```python
from build123d import *

# Parameters (mm, degrees)
SKETCH_2_R          = 2.25
CUT_EXTRUDE_1_DEPTH = 57.577380639
SKETCH_3_R          = 3.75
CUT_EXTRUDE_2_DEPTH = 4


with BuildPart() as part:
    # Эскиз1 → Повернуть1 (revolve)
    with BuildSketch(Plane.XY, mode=Mode.PRIVATE) as revolve_1_sk:
        Polygon((5, 55), (5, 0), (20, 0), (20, 6), (9.5, 6), (9.5, 55), align=None)
    revolve(revolve_1_sk.sketch.rotate(Axis((0, 53.580953173, 0), (0, -1, 0)), 90), axis=Axis((0, 53.580953173, 0), (0, -1, 0)))

    # Эскиз2 → Вырез-Вытянуть1 (cut, through all)
    with BuildSketch(Plane(origin=(0, 6, 0), x_dir=(1, 0, 0), z_dir=(0, 1, 0))):
        with Locations(Location((14.5, 0, 0), (0, 0, 270))):
            Circle(SKETCH_2_R)
        with Locations(Location((0, -14.5, 0), (0, 0, 270))):
            Circle(SKETCH_2_R)
        with Locations(Location((-14.5, 0, 0), (0, 0, 270))):
            Circle(SKETCH_2_R)
        with Locations(Location((0, 14.5, 0), (0, 0, 270))):
            Circle(SKETCH_2_R)
    extrude(amount=-CUT_EXTRUDE_1_DEPTH, mode=Mode.SUBTRACT)

    # Эскиз3 → Вырез-Вытянуть2 (cut)
    with BuildSketch(Plane.XZ):
        with Locations(Location((-14.5, 0, 0), (0, 0, 270))):
            Circle(SKETCH_3_R)
        with Locations(Location((0, 14.5, 0), (0, 0, 270))):
            Circle(SKETCH_3_R)
        with Locations(Location((14.5, 0, 0), (0, 0, 270))):
            Circle(SKETCH_3_R)
        with Locations(Location((0, -14.5, 0), (0, 0, 270))):
            Circle(SKETCH_3_R)
    extrude(amount=-CUT_EXTRUDE_2_DEPTH, mode=Mode.SUBTRACT)


solid = part.part
```
Could you check a few things on this model? Use its own coordinates, in mm. A direction names the side the tool comes from. Round coordinates to 2 decimals unless told otherwise and drop trailing zeros. Loops run counter-clockwise (first coordinate to the right, second up) from the corner with the lowest first, then second, coordinate; pieces in that order, holes last.
Q1. For P1, Ø6, axis at x = -14.5, z = 0, coming from the -Y side; P2, Ø8, axis at x = 11.5, y = 24, coming from the +Z side; P3, Ø3, axis at x = -3.5, y = 23, coming from the -Z side; P4, Ø12, axis at x = 0, z = 14.5, coming from the +Y side, each with a flat end and sliding along its axis, tell me the tip position at first contact or that it passes through.
Q2. I want a section at C-C (z = -15). Write out the boundary of the cut face in (x, y).
Q3. I want a section at B-B (x = 15.5). Write out the boundary of the cut face in (y, z), and give its area (3 significant figures).
Q4. Please list where these lines run through material, in increasing order: L1, parallel to X at y = 2.2, z = 0; L2, parallel to X at y = 4.4, z = 0; L3, parallel to X at y = 32, z = 0.
Q5. I want a section at A-A (z = 0). Write out the boundary of the cut face in (x, y).
Q6. On a 3-axis mill with a long thin cutter (end or side, diameter ignored), from which of +Z, -Z, +X, -X, +Y, -Y can I reach the whole of each face in a straight line? I mean faces 1 (the flat face through (-2, 4, 13)), 2 (the cylindrical face through (0, 27, -5)), 3 (the cylindrical face through (9.274, 30.843, -2.059)). Say none if no direction works.
Q7. Thinking about a two-plate mould opening in X: for faces 4 (the cylindrical face through (-0.88, 3.04, -19.98)), 5 (the flat face through (13, 4, -2)), 6 (the flat face through (4, 6, 9)), which applies, pulls with the +X half, pulls with the -X half, needs draft (parallel to the pull), parting line crosses it, or undercut?
Q8. I want a section at D-D (x = 0). Write out the boundary of the cut face in (y, z).
Answer below:
1. P1: stops at y = 4
1. P2: stops at z = 5.83
1. P3: stops at z = -9.29
1. P4: stops at y = 55
2. outline: (-13.23, 0) - (-3.72, 0) - (-3.72, 4) - (-2.19, 4) - (-2.19, 6) - (-13.23, 6) - close; (2.19, 4) - (3.72, 4) - (3.72, 0) - (13.23, 0) - (13.23, 6) - (2.19, 6) - close
3. outline: (0, -12.64) - (6, -12.64) - (6, -2.02) - (4, -2.02) - (4, -3.61) - (0, -3.61) - close; (0, 3.61) - (4, 3.61) - (4, 2.02) - (6, 2.02) - (6, 12.64) - (0, 12.64) - close
3. area: 115 mm2
4. L1: x = -20 to -18.25, -10.75 to -5, 5 to 10.75, 18.25 to 20
4. L2: x = -20 to -16.75, -12.25 to -5, 5 to 12.25, 16.75 to 20
4. L3: x = -9.5 to -5, 5 to 9.5
5. outline: (-20, 0) - (-18.25, 0) - (-18.25, 4) - (-16.75, 4) - (-16.75, 6) - (-20, 6) - close; (-12.25, 4) - (-10.75, 4) - (-10.75, 0) - (-5, 0) - (-5, 55) - (-9.5, 55) - (-9.5, 6) - (-12.25, 6) - close; (5, 0) - (10.75, 0) - (10.75, 4) - (12.25, 4) - (12.25, 6) - (9.5, 6) - (9.5, 55) - (5, 55) - close; (16.75, 4) - (18.25, 4) - (18.25, 0) - (20, 0) - (20, 6) - (16.75, 6) - close
6. face 1: -Y
6. face 2: +Y, -Y
6. face 3: +Y
7. face 4: parting line crosses it
7. face 5: undercut
7. face 6: needs draft
8. outline: (0, -20) - (6, -20) - (6, -16.75) - (4, -16.75) - (4, -18.25) - (0, -18.25) - close; (0, -10.75) - (4, -10.75) - (4, -12.25) - (6, -12.25) - (6, -9.5) - (55, -9.5) - (55, -5) - (0, -5) - close; (0, 5) - (55, 5) - (55, 9.5) - (6, 9.5) - (6, 12.25) - (4, 12.25) - (4, 10.75) - (0, 10.75) - close; (0, 18.25) - (4, 18.25) - (4, 16.75) - (6, 16.75) - (6, 20) - (0, 20) - close
